```python
from build123d import *

# Parameters (mm, degrees)
BOSS_EXTRUDE1_DEPTH            = 6.25
CHAMFER1_SIZE                  = 5
F_3_7_3_7_DIAMETER_HOLE1_D     = 3.7
F_3_7_3_7_DIAMETER_HOLE1_DEPTH = 12
F_3_7_3_7_DIAMETER_HOLE1_TIP   = 1.111592145
F_3_7_3_7_DIAMETER_HOLE2_D     = 3.7
F_3_7_3_7_DIAMETER_HOLE2_DEPTH = 20
F_3_7_3_7_DIAMETER_HOLE2_TIP   = 1.111592145


with BuildPart() as part:
    # Sketch1 → Boss-Extrude1 (new, symmetric)
    with BuildSketch(Plane(origin=(0, 0, 0), x_dir=(0, 0, -1), z_dir=(1, 0, 0))):
        Polygon((0, 0), (-17.045, 0), (-17.045, 61), (-53, 61), (-53, 96), (0, 96), align=None)
    extrude(amount=BOSS_EXTRUDE1_DEPTH, both=True)

    # Chamfer1
    chamfer1_edges = [part.edges().sort_by_distance(p)[0] for p in [
        (0, 61, 17.045),
        (0, 96, 0),
    ]]
    chamfer(chamfer1_edges, length=CHAMFER1_SIZE)

    # Ø3.7 (3.7) Diameter Hole1
    with Locations(Plane.XY.offset(53)):
        with Locations((0, 86), (0, 71)):
            Hole(F_3_7_3_7_DIAMETER_HOLE1_D / 2, depth=F_3_7_3_7_DIAMETER_HOLE1_DEPTH)
            with Locations((0, 0, -(F_3_7_3_7_DIAMETER_HOLE1_DEPTH + F_3_7_3_7_DIAMETER_HOLE1_TIP / 2))):  # 118° drill point
                Cone(0, F_3_7_3_7_DIAMETER_HOLE1_D / 2, F_3_7_3_7_DIAMETER_HOLE1_TIP, mode=Mode.SUBTRACT)

    # Ø3.7 (3.7) Diameter Hole2
    with Locations(Plane(origin=(0, 0, 0), x_dir=(-1, 0, 0), z_dir=(0, -1, 0))):
        with Locations((0, -10.22)):
            Hole(F_3_7_3_7_DIAMETER_HOLE2_D / 2, depth=F_3_7_3_7_DIAMETER_HOLE2_DEPTH)
            with Locations((0, 0, -(F_3_7_3_7_DIAMETER_HOLE2_DEPTH + F_3_7_3_7_DIAMETER_HOLE2_TIP / 2))):  # 118° drill point
                Cone(0, F_3_7_3_7_DIAMETER_HOLE2_D / 2, F_3_7_3_7_DIAMETER_HOLE2_TIP, mode=Mode.SUBTRACT)


solid = part.part
```
Can you work these out from the model? Positions are in its coordinate system, mm. A direction names the side the tool comes from. Give positions to 0.01 mm unless a question says otherwise; leave off trailing zeros. Loops run counter-clockwise (first coordinate to the right, second up) from the corner with the lowest first, then second, coordinate; pieces in that order, holes last. Notation, with made-up numbers: M -37.5,-32 L 2.5,-32 A20 cw 2.5,0 Z; hole C 46.5,-8.5 d11. An arc over 180 degrees is marked long. Use one line per item in the form item = value. Start each with the question number.
(1) I'm going to push a flat-ended pin straight in: P1, Ø4, axis at x = 3, y = 39, coming from the +Z side (3 decimals). Where does the tip first touch, or does it pass through?
(2) I want a section at C-C, the plane z = 46. Write out the boundary of the cut face in (x, y), and give its area (3 significant figures).
(3) I want a section at D-D, the plane z = 30. Write out the boundary of the cut face in (x, y).
(4) On a 3-axis mill with a long thin cutter (end or side, diameter ignored), from which of +Z, -Z, +X, -X, +Y, -Y can I reach the whole of each face in a straight line? I mean faces 1 (the cylindrical face through (1.765, 10.14, 9.664)), 2 (the cylindrical face through (0.401, 69.194, 46.916)), 3 (the flat face through (0, 61, 37)). Say none if no direction works.
(5) I want a section at A-A, the plane x = -5. Write out the boundary of the cut face in (y, z) (3 decimals).
(6) Thinking about a two-plate mould opening in X: for faces 4 (the flat face through (1, 0, 8)), 5 (the cylindrical face through (0.401, 84.194, 46.916)), 6 (the flat face through (-6.25, 59, 14)), which applies, released by +X, released by -X, zero draft, split by the parting line, or undercut?
(7) Please list where these lines run through material, in increasing order: line 1 (Y direction, x = 0, z = 44.5); line 2 (X direction, y = 71, z = 47); line 3 (Z direction, x = 5.25, y = 47.5) (3 decimals).
(8) I want a section at B-B, the plane y = 19. Write out the boundary of the cut face in (x, z) (3 decimals), and give its area (3 significant figures).
Worked out:
q1.P1 = 17.045
q2.outline = M -6.25,61 L 6.25,61 L 6.25,96 L -6.25,96 Z; hole C 0,71 d3.7; hole C 0,86 d3.7
q2.area = 416 mm²
q3.outline = M -6.25,61 L 6.25,61 L 6.25,96 L -6.25,96 Z
q4.face_1 = -Y
q4.face_2 = +Z
q4.face_3 = +Z, +X, -X, -Y
q5.outline = M 0,0 L 91,0 L 96,5 L 96,53 L 61,53 L 61,22.045 L 56,17.045 L 0,17.045 Z
q6.face_4 = zero draft
q6.face_5 = undercut
q6.face_6 = released by -X
q7.line_1 = 61 to 69.15, 72.85 to 84.15, 87.85 to 96
q7.line_2 = -6.25 to -1.85, 1.85 to 6.25
q7.line_3 = 0 to 17.045
q8.outline = M -6.25,0 L 6.25,0 L 6.25,17.045 L -6.25,17.045 Z; hole C 0,10.22 d3.7
q8.area = 202 mm²
